Check sheet for the modelled part. Datum: model origin and axes. Units: mm. Face numbers are marked on the shaded views. A direction names the side the tool comes from. Round coordinates to 2 decimals unless told otherwise and drop trailing zeros. Loops run counter-clockwise (first coordinate to the right, second up) from the corner with the lowest first, then second, coordinate; pieces in that order, holes last. Notation, with made-up numbers: M 7.25,40 L 53.25,40 A31 ccw 53.25,78 Z; hole C -28,35 d9. An arc over 180 degrees is marked long. One line per question, with ' | ' between items. Start each with the question number.
(1) Draft check along Z on the marked faces 6, 7, 8 and 9. Enter one of: +Z half, -Z half, draft (parallel to the pull), parting line (faces both ways), or undercut.
(2) Tool access check on the marked faces 1, 2, 3, 4 and 5. Record the directions out of +Z, -Z, +X, -X, +Y, -Y that give a thin tool (end or side, any length) a straight path to the whole face; none if there is none.
(3) Thickness scan on probe 1 along X at (y, z) = (8.5, 0); probe 2 along Z at (x, y) = (-8.5, 2.5); probe 3 along Z at (x, y) = (10, 6). Record the ranges inside material, lowest first. Write a range as [from, to].
(4) Section check B-B (y = 2.25). Record the boundary of the cut face in (x, z), and give its area (3 significant figures).
(5) Section check C-C (x = 0). Record the boundary of the cut face in (y, z).
(6) Section check D-D (y = 7.25). Record the boundary of the cut face in (x, z).
(7) Section check A-A (x = 10). Record the boundary of the cut face in (y, z), and give its area (3 significant figures).
(8) Go/stop test with flat-tipped pins: P1, Ø10, axis at x = -26, z = -16.5, coming from the +Y side; P2, Ø11, axis at x = -2.5, z = 0, coming from the +Y side; P3, Ø4, axis at x = 0.5, z = -31.5, coming from the +Y side; P4, Ø6, axis at x = 10, z = 0, coming from the -Y side. Record where each tip stops, or that it passes through.
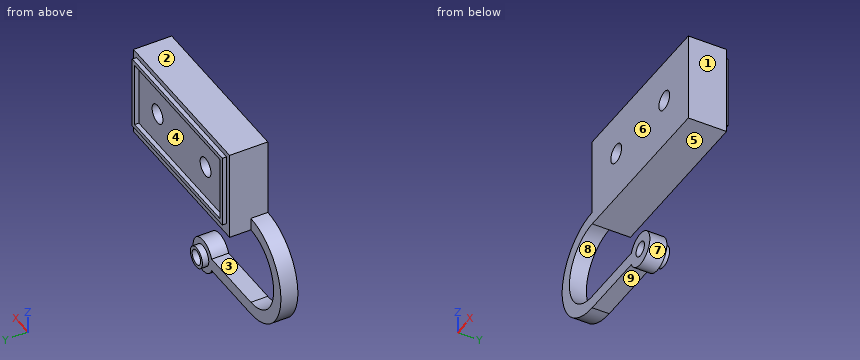
```python
from build123d import *

# Parameters (mm, degrees)
SKETCH1_W           = 40
SKETCH1_H           = 18.5
SKETCH1_R           = 2.25
SKETCH1_H_2         = 1.5
BOSS_EXTRUDE3_DEPTH = 9
SKETCH1_5_R         = 1.75
BOSS_EXTRUDE4_DEPTH = 4
SKETCH2_R           = 2.5
SKETCH2_R_2         = 1.75
BOSS_EXTRUDE5_DEPTH = 1.5
SKETCH3_W           = 37.5
SKETCH3_H           = 17.5
SKETCH3_W_2         = 35.5
SKETCH3_H_2         = 15.5
BOSS_EXTRUDE6_DEPTH = 1


with BuildPart() as part:
    # Sketch1 → Boss-Extrude3 (new body)
    with BuildSketch(Plane(origin=(0, 0, 0), x_dir=(1, 0, 0), z_dir=(0, 1, 0))):
        with Locations((0, -0.75)):
            Rectangle(SKETCH1_W, SKETCH1_H)
        with Locations((-10, 0)):
            Circle(SKETCH1_R, mode=Mode.SUBTRACT)
        with Locations((10, 0)):
            Circle(SKETCH1_R, mode=Mode.SUBTRACT)
        with Locations((0, 10.75)):
            Rectangle(SKETCH1_W, SKETCH1_H_2)
        with Locations((0, 9.25)):
            Rectangle(SKETCH1_W, SKETCH1_H_2)
    extrude(amount=BOSS_EXTRUDE3_DEPTH)

    # Sketch1_5 → Boss-Extrude4 (add)
    with BuildSketch(Plane(origin=(0, 0, 0), x_dir=(1, 0, 0), z_dir=(0, 1, 0))):
        with BuildLine():
            ThreePointArc((-20, 33.5), (-32.5, 21), (-20, 8.5))
            Line((-20, 8.5), (-20, 10))
            Line((-20, 10), (-20, 11.5))
            ThreePointArc((-20, 11.5), (-29.5, 21), (-20, 30.5))
            Line((-20, 30.5), (-3.708099244, 30.5))
            ThreePointArc((-3.708099244, 30.5), (4, 32), (-3.708099244, 33.5))
            Line((-3.708099244, 33.5), (-20, 33.5))
        make_face()
        with Locations((0, 32)):
            Circle(SKETCH1_5_R, mode=Mode.SUBTRACT)
    extrude(amount=BOSS_EXTRUDE4_DEPTH)

    # Sketch2 → Boss-Extrude5 (add)
    with BuildSketch(Plane(origin=(0, 4, 0), x_dir=(1, 0, 0), z_dir=(0, 1, 0))):
        with Locations((0, 32)):
            Circle(SKETCH2_R)
        with Locations((0, 32)):
            Circle(SKETCH2_R_2, mode=Mode.SUBTRACT)
    extrude(amount=BOSS_EXTRUDE5_DEPTH)

    # Sketch3 → Boss-Extrude6 (add)
    with BuildSketch(Plane(origin=(0, 9, 0), x_dir=(1, 0, 0), z_dir=(0, 1, 0))):
        Rectangle(SKETCH3_W, SKETCH3_H)
        Rectangle(SKETCH3_W_2, SKETCH3_H_2, mode=Mode.SUBTRACT)
    extrude(amount=BOSS_EXTRUDE6_DEPTH)


solid = part.part
```
The answers:
1) face 6: draft | face 7: undercut | face 8: undercut | face 9: -Z half
2) face 1: +Z, -Z, +X, +Y, -Y | face 2: +Z, +X, -X, +Y, -Y | face 3: +Y, -Y | face 4: +Y | face 5: +X, +Y, -Y
3) probe 1: [-20, -12.25], [-7.75, 7.75], [12.25, 20] | probe 2: [-33.5, -30.5], [-11.5, -1.68], [1.68, 10] | probe 3: [-11.5, -2.25], [2.25, 10]
4) outline: M -20,-33.5 L -3.71,-33.5 A4 ccw long -3.71,-30.5 L -20,-30.5 A9.5 cw -20,-11.5 L 20,-11.5 L 20,10 L -20,10 L -20,-8.5 A12.5 ccw Z; hole C -10,0 d4.5; hole C 0,-32 d3.5; hole C 10,0 d4.5 | area: 1,020 mm²
5) outline: M 0,-36 L 4,-36 L 4,-34.5 L 5.5,-34.5 L 5.5,-33.75 L 0,-33.75 Z; M 0,-30.25 L 5.5,-30.25 L 5.5,-29.5 L 4,-29.5 L 4,-28 L 0,-28 Z; M 0,-11.5 L 9,-11.5 L 9,-8.75 L 10,-8.75 L 10,-7.75 L 9,-7.75 L 9,7.75 L 10,7.75 L 10,8.75 L 9,8.75 L 9,10 L 0,10 Z
6) outline: M -20,-11.5 L 20,-11.5 L 20,10 L -20,10 Z; hole C -10,0 d4.5; hole C 10,0 d4.5
7) outline: M 0,-11.5 L 9,-11.5 L 9,-8.75 L 10,-8.75 L 10,-7.75 L 9,-7.75 L 9,-2.25 L 0,-2.25 Z; M 0,2.25 L 9,2.25 L 9,7.75 L 10,7.75 L 10,8.75 L 9,8.75 L 9,10 L 0,10 Z | area: 155 mm²
8) P1: y = 4 | P2: y = 9 | P3: y = 5.5 | P4: y = 0
